Part print with two shaded views. Sizes in mm from the minimum x, y, z corner. Round coordinates to 2 decimals unless told otherwise and drop trailing zeros. Loops run counter-clockwise (first coordinate to the right, second up) from the corner with the lowest first, then second, coordinate; pieces in that order, holes last. Notation, with made-up numbers: (21, 54) - (75, 54) arc R12 ccw to (75, 63) - close; hole circle Ø10 at (31.25, 79). An arc over 180 degrees is marked (long way). Use a Markdown table: item, result.
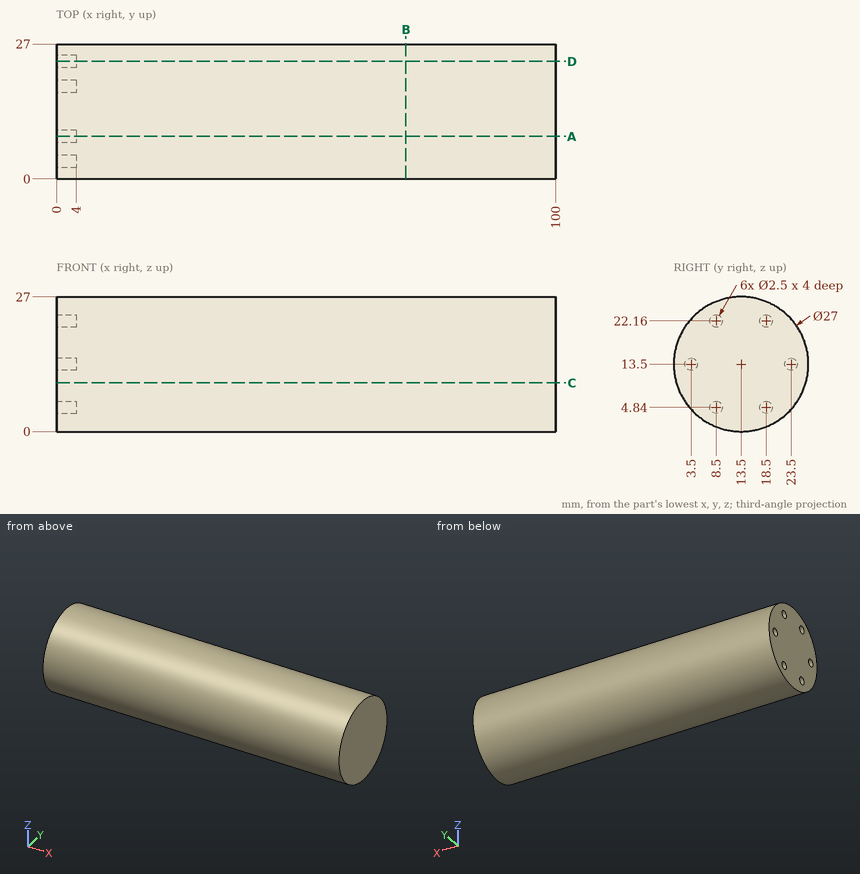
Q1. Drop flat-ended pins along their axis: pin 1 (1.5 mm diameter, centred on y = 23.5, z = 13.5, fed in from -X); pin 2 (10 mm diameter, centred on x = 10.5, z = 3.5, fed in from -Y); pin 3 (10 mm diameter, centred on x = 40, z = 20.5, fed in from -Y). Give the stop position or say it passes through.
Results found:
| item | result |
|---|---|
| pin 1 | stops at x = 4 |
| pin 2 | stops at y = 0.96 |
| pin 3 | stops at y = 0.15 |
Q2. Cut at B-B, the plane x = 70. List the corners of the cut face in (y, z).
Results found:
| item | result |
|---|---|
| outline | circle Ø27 at (13.5, 13.5) |
Q3. Cut at A-A, the plane y = 8.5. List the corners of the cut face in (x, z).
Results found:
| item | result |
|---|---|
| outline | (0, 0.96) - (100, 0.96) - (100, 26.04) - (0, 26.04) - (0, 23.41) - (4, 23.41) - (4, 20.91) - (0, 20.91) - (0, 6.09) - (4, 6.09) - (4, 3.59) - (0, 3.59) - close |
Q4. Cut at D-D, the plane y = 23.5. List the corners of the cut face in (x, z).
Results found:
| item | result |
|---|---|
| outline | (0, 4.43) - (100, 4.43) - (100, 22.57) - (0, 22.57) - (0, 14.75) - (4, 14.75) - (4, 12.25) - (0, 12.25) - close |
Q5. Probe line 1 (Y direction, x = 1.75, z = 13.5); line 2 (Y direction, x = 39.5, z = 6.5); line 3 (Z direction, x = 89, y = 17.75). List the from-to ranges inside material, lowest first.
Results found:
| item | result |
|---|---|
| line 1 | y = 0 to 2.25, 4.75 to 22.25, 24.75 to 27 |
| line 2 | y = 1.96 to 25.04 |
| line 3 | z = 0.69 to 26.31 |
Q6. Cut at C-C, the plane z = 9.75. List the corners of the cut face in (x, y), plus the area to 3 significant figures.
Results found:
| item | result |
|---|---|
| outline | (0, 0.53) - (100, 0.53) - (100, 26.47) - (0, 26.47) - close |
| area | 2,590 mm2 |
